Design review of the part shown in the three views and the two pictorial views. Dimensions are in mm from the part's minimum x, y and z. Coordinates: 2 decimals unless noted, no trailing zeros. Write each loop counter-clockwise with the first axis right and the second up, starting at its lowest first coordinate (ties: lowest second). Pieces come first, ordered by that corner, then holes. Notation, with made-up numbers: (27.25, -38.5) -> (76.25, -38.5) arc R14 cw to (76.25, -25.5) -> close; hole circle Ø1 at (60.5, 77). An arc over 180 degrees is marked (long way). Write item = value, one per line. Start each with the question number.
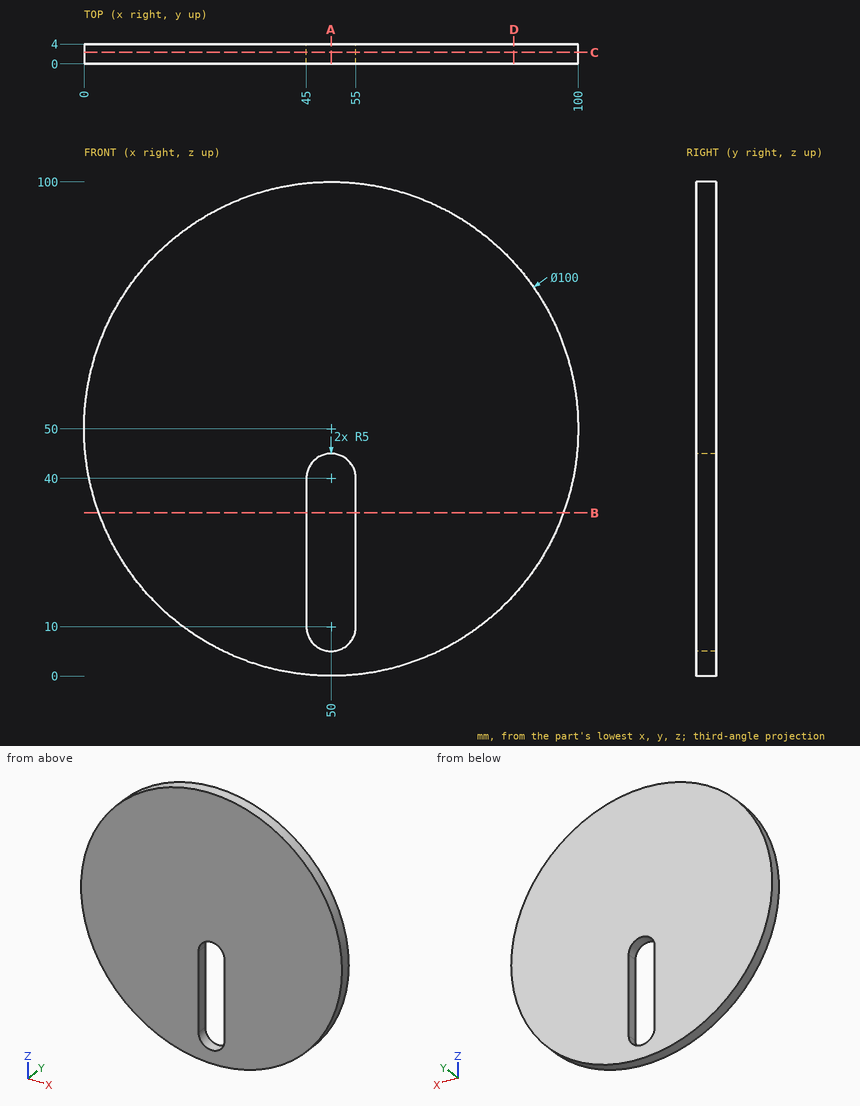
(1) Take a section at D-D, the plane x = 87. State the section outline as (y, z) points, then the cut area to 3 significant figures.
(2) For line 1 (X direction, y = 0.85, z = 51); line 2 (X direction, y = 3.35, z = 15.5); line 3 (X direction, y = 0.85, z = 75.5), list the stretches that pass through material, from the lowest coordinate up.
(3) Take a section at B-B, the plane z = 33. State the section outline as (x, y) points.
(4) Take a section at C-C, the plane y = 2.3. State the section outline as (x, z) points.
(5) Take a section at A-A, the plane x = 50. State the section outline as (y, z) points, then the cut area to 3 significant figures.
(6) For pin 1 Ø1 at (y, z) = (3, 30.5) entering from +X; pin 2 Ø1.5 at (y, z) = (3, 26.5) entering from -X; pin 3 Ø2 at (y, z) = (1.5, 20) entering from -X, all flat-tipped, find the tip position at first contact; note any pin that passes through.
Report:
q1.outline = (0, 16.37) -> (4, 16.37) -> (4, 83.63) -> (0, 83.63) -> close
q1.area = 269 mm2
q2.line_1 = 0.01 to 99.99
q2.line_2 = 13.81 to 45, 55 to 86.19
q2.line_3 = 6.99 to 93.01
q3.outline = (2.98, 0) -> (45, 0) -> (45, 4) -> (2.98, 4) -> close; (55, 0) -> (97.02, 0) -> (97.02, 4) -> (55, 4) -> close
q4.outline = circle Ø100 at (50, 50); hole (45, 10) arc R5 ccw to (55, 10) -> (55, 40) arc R5 ccw to (45, 40) -> close
q5.outline = (0, 0) -> (4, 0) -> (4, 5) -> (0, 5) -> close; (0, 45) -> (4, 45) -> (4, 100) -> (0, 100) -> close
q5.area = 240 mm2
q6.pin_1 = 96.25
q6.pin_2 = 5.48
q6.pin_3 = 9.27
